Autodesk Inventor part; units mm, degrees
ref_plane "YZ Plane" through (0, 0, 0) normal (1, 0, 0) x (0, 1, 0)
ref_plane "XZ Plane" through (0, 0, 0) normal (0, 1, 0) x (-1, 0, 0)
ref_plane "XY Plane" through (0, 0, 0) normal (0, 0, 1) x (1, 0, 0)
sketch "Sketch1" plane through (0, 0, 0) normal (0, 0, 1) x (1, 0, 0)
  line L0 (0, 0) -> (0, 3.85)
  line L1 (0, 0) -> (19.15, 0)
  line L2 (19.15, 0) -> (19.15, 3.85)
  line L3 (0, 3.85) -> (2.325, 3.85)
  line L4 (2.325, 3.85) -> (2.325, 6)
  line L5 (19.15, 3.85) -> (16.825, 3.85)
  line L6 (16.825, 3.85) -> (16.825, 6)
  arc A0 (16.825, 6) -> (2.325, 6) centre (9.575, 6) ccw
  circle A1 centre (9.575, 6.12) radius 3.7
  point P0 (9.575, 13.25)
  dimension "d0" = 19.15
  dimension "d1" = 3.85
  dimension "d2" = 3.85
  dimension "d3" = 9.575
  dimension "d4" = 13.25
  dimension "d5" = 7.25
  dimension "d6" = 7.25
  dimension "d7" = 7.25
  dimension "d8" = 7.25
  dimension "d9" = 9.575
  dimension "d10" = 7.4
  dimension "d11" = 7.13
extrude "Extrusion1" add sketch "Sketch1" along normal blind 6
fillet "Fillet1" radius 1.5 2 edges at (19.15, 1.925, 0) (0, 1.925, 0)
equation "\"d2\" = d1"
equation "\"d9\" = d3"
properties part number "Recoil Spring Mount v1.0"
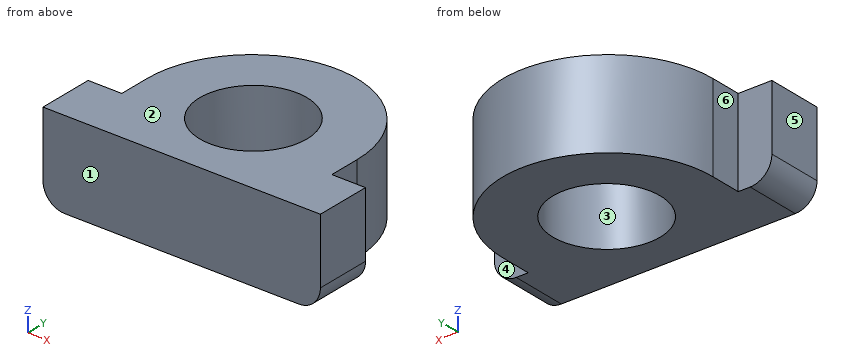
Read the model definition and answer for the solid it produces. Units are mm, in the model's axes. Face numbers are marked on the shaded views. A direction names the side the tool comes from. Round coordinates to 2 decimals unless told otherwise and drop trailing zeros. Write each loop counter-clockwise with the first axis right and the second up, starting at its lowest first coordinate (ties: lowest second). Pieces come first, ordered by that corner, then holes. Notation, with made-up numbers: (-6, -35) -> (25, -35) arc R20 cw to (25, -9) -> close; hole circle Ø3 at (-16.5, 71). An arc over 180 degrees is marked (long way). Answer in a Markdown table with one row per item. Add a question column.
1) Find section B-B, the plane y = 8.25. Determine the outline of the cut face in (x, z).
2) Which of the six approach directions +Z, -Z, +X, -X, +Y, -Y give full straight-line access (tool end or side, diameter ignored) to the marked faces 5 and 6?
3) Determine the mould class of the marked faces 1, 2, 3 and 4 for opening direction Y: pulls with the +Y half, pulls with the -Y half, needs draft (parallel to the pull), parting line crosses it, or undercut.
4) Find section D-D, the plane y = 3. Determine the outline of the cut face in (x, z).
5) Given P1, Ø1.1, axis at y = 5, z = 4, coming from the -X side (3 decimals); P2, Ø0.6, axis at y = 5, z = 3.5, coming from the +X side (3 decimals); P3, Ø3, axis at x = 12, z = 1.5, coming from the +Y side, each flat-ended and moving along its own axis, determine where each tip first touches the part or whether it passes through.
6) Find section A-A, the plane z = 4. Determine the outline of the cut face in (x, y) (3 decimals), and give its area (3 significant figures).
7) Consider line 1 (Y direction, x = 17.5, z = 0.55); line 2 (X direction, y = 3, z = 2.3); line 3 (X direction, y = 5, z = 4.2) (3 decimals). Determine where each line is inside the solid, lowest interval first.
8) Find section C-C, the plane x = 12. Determine the outline of the cut face in (y, z).
Findings below:
| question | item | result |
|---|---|---|
| 1 | outline | (2.68, 0) -> (6.55, 0) -> (6.55, 6) -> (2.68, 6) -> close; (12.6, 0) -> (16.47, 0) -> (16.47, 6) -> (12.6, 6) -> close |
| 2 | face 5 | +Z, -Z, -X, +Y, -Y |
| 2 | face 6 | +Z, -Z, -X, +Y |
| 3 | face 1 | pulls with the -Y half |
| 3 | face 2 | needs draft |
| 3 | face 3 | undercut |
| 3 | face 4 | pulls with the +Y half |
| 4 | outline | (0, 1.5) arc R1.5 ccw to (1.5, 0) -> (7.59, 0) -> (7.59, 6) -> (0, 6) -> close; (11.56, 0) -> (17.65, 0) arc R1.5 ccw to (19.15, 1.5) -> (19.15, 6) -> (11.56, 6) -> close |
| 5 | P1 | x = 2.325 |
| 5 | P2 | x = 16.825 |
| 5 | P3 | y = 13.19 |
| 6 | outline | (0, 0) -> (19.15, 0) -> (19.15, 3.85) -> (16.825, 3.85) -> (16.825, 6) arc R7.25 ccw to (2.325, 6) -> (2.325, 3.85) -> (0, 3.85) -> close; hole circle Ø7.4 at (9.575, 6.12) |
| 6 | area | 144 mm² |
| 7 | line 1 | 0 to 3.85 |
| 7 | line 2 | 0 to 7.59, 11.56 to 19.15 |
| 7 | line 3 | 2.325 to 6.049, 13.101 to 16.825 |
| 8 | outline | (0, 0) -> (3.33, 0) -> (3.33, 6) -> (0, 6) -> close; (8.91, 0) -> (12.83, 0) -> (12.83, 6) -> (8.91, 6) -> close |
